from build123d import *

# Parameters (mm, degrees)
BATTERY_REMOVABLE_CLAMP_BAR_START = 43
SKETCH_1_W                        = 90
SKETCH_1_H                        = 10
BATTERY_REMOVABLE_CLAMP_BAR_DEPTH = 4
CLAMP_TWO_M3_START                = 48
SKETCH_2_R                        = 1.7
CLAMP_TWO_M3_DEPTH                = 6


with BuildPart() as part:
    # 草图1 → Battery_removable_clamp_bar (new body)
    with BuildSketch(Plane.XY.offset(BATTERY_REMOVABLE_CLAMP_BAR_START)):
        with Locations((6, 0)):
            Rectangle(SKETCH_1_W, SKETCH_1_H)
    extrude(amount=BATTERY_REMOVABLE_CLAMP_BAR_DEPTH)

    # 草图2 → Clamp_two_M3 (cut)
    with BuildSketch(Plane.XY.offset(CLAMP_TWO_M3_START)):
        with Locations(Location((-35, 0, 0), (0, 0, 180))):
            Circle(SKETCH_2_R)
        with Locations(Location((47, 0, 0), (0, 0, 180))):
            Circle(SKETCH_2_R)
    extrude(amount=-CLAMP_TWO_M3_DEPTH, mode=Mode.SUBTRACT)


solid = part.part
Geometry: final body of the model. Coordinates: model frame, mm. Round coordinates to 2 decimals unless told otherwise and drop trailing zeros. Loops run counter-clockwise (first coordinate to the right, second up) from the corner with the lowest first, then second, coordinate; pieces in that order, holes last.
Q1. Pin query (flat end, axial travel): P1, Ø3, axis at x = 47, y = 0, coming from the +Z side. Return the tip coordinate at first contact, or that it passes through.
Q2. Pull-direction query (X, two-part tool) for faces 1 (the cylindrical face through (-33.65, 1.03, 45.03)), 2 (the flat face through (5, 0, 43)), 3 (the flat face through (51, 0, 45)); classes: released by +X, released by -X, zero draft, split by the parting line, or undercut.
Q3. Section A-A on y = 0. Return loops of the section in (x, z).
Q4. Section B-B on x = -35. Return loops of the section in (y, z).
Q5. Material intervals for L1, parallel to X at y = -0.25, z = 45.5; L2, parallel to Y at x = -35, z = 44.7; L3, parallel to X at y = 1.5, z = 45.65, sorted ascending.
Evaluation:
1. P1: passes through
2. face 1: undercut
2. face 2: zero draft
2. face 3: released by +X
3. outline: (-39, 43) - (-36.7, 43) - (-36.7, 47) - (-39, 47) - close; (-33.3, 43) - (45.3, 43) - (45.3, 47) - (-33.3, 47) - close; (48.7, 43) - (51, 43) - (51, 47) - (48.7, 47) - close
4. outline: (-5, 43) - (-1.7, 43) - (-1.7, 47) - (-5, 47) - close; (1.7, 43) - (5, 43) - (5, 47) - (1.7, 47) - close
5. L1: x = -39 to -36.68, -33.32 to 45.32, 48.68 to 51
5. L2: y = -5 to -1.7, 1.7 to 5
5. L3: x = -39 to -35.8, -34.2 to 46.2, 47.8 to 51
